from build123d import *

# Parameters (mm, degrees)
SKETCH_1_W          = 36
SKETCH_1_H          = 26
EXTRUDE_1_DEPTH     = 6
EXTRUDE_START       = -5
EXTRUDE_2_DEPTH     = 10
SKETCH_3_R          = 1.6
CUT_EXTRUDE_2_DEPTH = 70.491006612
SKETCH_4_R          = 3
CUT_EXTRUDE_3_DEPTH = 70.491006612


with BuildPart() as part:
    # 草图1 → 凸台-拉伸1 (new body)
    with BuildSketch(Plane.XY):
        with Locations((18, 0)):
            Rectangle(SKETCH_1_W, SKETCH_1_H)
    extrude(amount=EXTRUDE_1_DEPTH)

    # 草图2 → 凸台-拉伸2 (add)
    with BuildSketch(Plane(origin=(0, 0, 0), x_dir=(1, 0, 0), z_dir=(0, 1, 0)).offset(EXTRUDE_START)):
        Polygon((8, -6), (28, -6), (28, -40), (24, -58), (12, -58), (8, -46), align=None)
    extrude(amount=EXTRUDE_2_DEPTH)

    # 草图3 → 切除-拉伸2 (cut, through all)
    with BuildSketch(Plane.XY):
        with Locations(Location((8, 0, 0), (0, 0, 90))):
            Circle(SKETCH_3_R)
        with Locations(Location((30, -9, 0), (0, 0, 180))):
            Circle(SKETCH_3_R)
        with Locations(Location((30, 9, 0), (0, 0, 180))):
            Circle(SKETCH_3_R)
        with Locations(Location((3, 0, 0), (0, 0, 180))):
            Circle(SKETCH_3_R)
    extrude(amount=CUT_EXTRUDE_2_DEPTH, mode=Mode.SUBTRACT)

    # 草图4 → 切除-拉伸3 (cut, through all)
    with BuildSketch(Plane(origin=(0, 0, 0), x_dir=(1, 0, 0), z_dir=(0, 1, 0))):
        with Locations(Location((18, -54, 0), (0, 0, 270))):
            Circle(SKETCH_4_R)
        with Locations(Location((18, -18, 0), (0, 0, 270))):
            Circle(SKETCH_4_R)
        with Locations(Location((18, -36, 0), (0, 0, 270))):
            Circle(SKETCH_4_R)
    extrude(amount=-CUT_EXTRUDE_3_DEPTH, mode=Mode.SUBTRACT)


solid = part.part
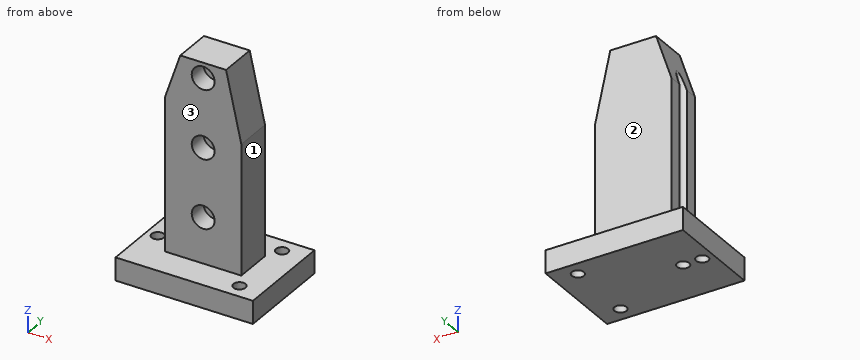
Build history of the part. All positions in model axes, mm. Face numbers are marked on the shaded views. A direction names the side the tool comes from. Give positions to 0.01 mm unless a question says otherwise; leave off trailing zeros. Loops run counter-clockwise (first coordinate to the right, second up) from the corner with the lowest first, then second, coordinate; pieces in that order, holes last. Notation, with made-up numbers: (51.25, 15.25) - (88.25, 15.25) arc R4 cw to (88.25, 20.25) - close; hole circle Ø10 at (-25, 87.25). An arc over 180 degrees is marked (long way). Write item = value, one per line. Start each with the question number.
1) Band-saw the part on C-C on x = 13.5. Give the cut face in (y, z).
2) Band-saw the part on B-B on x = 30. Give the cut face in (y, z).
3) Tool access for the marked faces 1, 2 and 3: list every direction of +Z, -Z, +X, -X, +Y, -Y with a clear straight run to the whole face (end or side of a thin tool).
4) Probe probe 1 along X at (y, z) = (-9, 4.15); probe 2 along X at (y, z) = (-2.2, 18); probe 3 along Y at (x, z) = (12, 56.5). List the from-to ranges inside material, lowest first. Write a range as from..to.
5) Drop flat-ended pins along their axis: pin 1 Ø8 at (x, z) = (18, 36) entering from -Y; pin 2 Ø5.5 at (x, z) = (18, 18) entering from -Y; pin 3 Ø1 at (y, z) = (2.5, 31.5) entering from -X; pin 4 Ø4 at (x, z) = (5, 42.5) entering from -Y. Give the stop position or say it passes through.
6) Band-saw the part on D-D on y = 1. Give the cut face in (x, z), plus the area to 3 significant figures.
7) Band-saw the part on A-A on y = -9. Give the cut face in (x, z), plus the area to 3 significant figures.
Final values:
q1.outline = (-13, 0) - (13, 0) - (13, 6) - (5, 6) - (5, 58) - (-5, 58) - (-5, 6) - (-13, 6) - close
q2.outline = (-13, 0) - (-10.6, 0) - (-10.6, 6) - (-13, 6) - close; (-7.4, 0) - (7.4, 0) - (7.4, 6) - (-7.4, 6) - close; (10.6, 0) - (13, 0) - (13, 6) - (10.6, 6) - close
q3.face_1 = +Z, +X, +Y, -Y
q3.face_2 = +Z, +X, -X, +Y
q3.face_3 = +Z, +X, -X, -Y
q4.probe_1 = 0..28.4, 31.6..36
q4.probe_2 = 8..15, 21..28
q4.probe_3 = -5..5
q5.pin_1 = -5
q5.pin_2 = 0
q5.pin_3 = 8
q5.pin_4 = through
q6.outline = (0, 0) - (1.75, 0) - (1.75, 6) - (0, 6) - close; (4.25, 0) - (6.75, 0) - (6.75, 6) - (4.25, 6) - close; (9.25, 0) - (36, 0) - (36, 6) - (28, 6) - (28, 40) - (24, 58) - (12, 58) - (9.25, 49.75) - close
q6.area = 1,110 mm²
q7.outline = (0, 0) - (28.4, 0) - (28.4, 6) - (0, 6) - close; (31.6, 0) - (36, 0) - (36, 6) - (31.6, 6) - close
q7.area = 197 mm²
